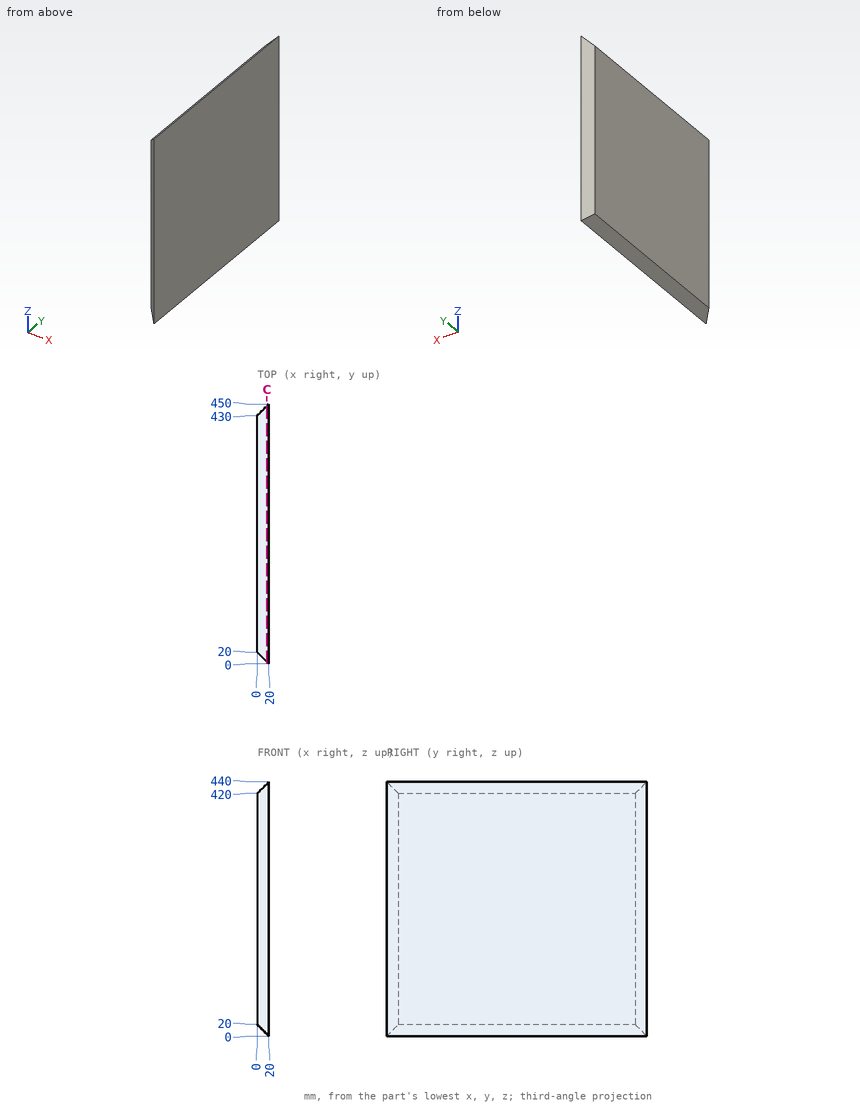
Drawing for the job (mm, zero at the part's lowest x, y, z). Give positions to 0.01 mm unless a question says otherwise; leave off trailing zeros. Order: outer loops, then holes, each group sorted by start corner. A loop starts at its lowest first (then second) coordinate and runs counter-clockwise, first axis right, second up. Notation, with made-up numbers: M 69.5,66 L 128.5,66 A19 ccw 128.5,82 Z; hole C -40,3.25 d3. An arc over 180 degrees is marked long. Put each result on its own line as item: value. Start each with the question number.
(1) Drill centre lines: line 1 along Z through (x, y) = (3.25, 101); line 2 along Y through (x, z) = (4.5, 284.5); line 3 along Y through (x, z) = (12, 63). Where is each one in solid material? Low to high.
(2) Saw through at C-C, the plane x = 16.75. Write the cut outline in (y, z).
(3) Flat gauge pins, fed straight in: pin 1 Ø1 at (x, z) = (3.5, 262.5) entering from -Y; pin 2 Ø2 at (x, z) = (5.5, 102.5) entering from +Y; pin 3 Ø5 at (x, z) = (14, 84.5) entering from -Y. Where does each tip first touch, or does it go through?
Check result:
1. line 1: z = 16.75 to 423.25
1. line 2: y = 15.5 to 434.5
1. line 3: y = 8 to 442
2. outline: M 3.25,3.25 L 446.75,3.25 L 446.75,436.75 L 3.25,436.75 Z
3. pin 1: stops at y = 16
3. pin 2: stops at y = 436.5
3. pin 3: stops at y = 3.5
